Check sheet for the modelled part. Datum: model origin and axes. Units: mm. Face numbers are marked on the shaded views. A direction names the side the tool comes from. Round coordinates to 2 decimals unless told otherwise and drop trailing zeros. Order: outer loops, then holes, each group sorted by start corner. A loop starts at its lowest first (then second) coordinate and runs counter-clockwise, first axis right, second up.
(1) Sectioned sample at B-B, the plane x = 0. Enter the section's corners in (y, z).
(2) Tool access check on the marked faces 1, 2, 3, 4 and 5. Record the directions out of +Z, -Z, +X, -X, +Y, -Y that give a thin tool (end or side, any length) a straight path to the whole face; none if there is none.
(3) Depth check by flat-ended pin: pin 1 (2 mm diameter, centred on x = -1, z = -1.5, fed in from -Y); pin 2 (0.6 mm diameter, centred on x = -0.5, y = 1, fed in from +Z). Enter the tip coordinate at first touch or a pass-through.
(4) Thickness scan on probe 1 along Z at (x, y) = (0.7, -1); probe 2 along Z at (x, y) = (-2.4, -3); probe 3 along Y at (x, z) = (2.1, 4). Record the ranges inside material, lowest first.
(5) Sectioned sample at C-C, the plane y = 1.75. Enter the section's corners in (x, z), and give its area (3 significant figures).
(6) Sectioned sample at A-A, the plane z = 0. Enter the section's corners in (x, y).
(7) Sectioned sample at D-D, the plane z = 2. Enter the section's corners in (x, y), and give its area (3 significant figures).
```python
from build123d import *

# Parameters (mm, degrees)
SKETCH1_W           = 6
SKETCH1_H           = 6.95
BOSS_EXTRUDE1_DEPTH = 1.95
SKETCH2_R           = 2.5
BOSS_EXTRUDE2_DEPTH = 1.7
SKETCH3_W           = 6
SKETCH3_H           = 0.5
BOSS_EXTRUDE3_DEPTH = 1
SKETCH4_W           = 6
SKETCH4_H           = 0.5
BOSS_EXTRUDE4_DEPTH = 6


with BuildPart() as part:
    # Sketch1 → Boss-Extrude1 (new, symmetric)
    with BuildSketch(Plane(origin=(0, 0, 0), x_dir=(1, 0, 0), z_dir=(0, 1, 0))):
        with Locations((0, -0.825)):
            Rectangle(SKETCH1_W, SKETCH1_H)
    extrude(amount=BOSS_EXTRUDE1_DEPTH, both=True)

    # Sketch2 → Boss-Extrude2 (add)
    with BuildSketch(Plane(origin=(0, 1.95, 0), x_dir=(1, 0, 0), z_dir=(0, 1, 0))):
        with Locations(Location((0, 0, 0), (0, 0, 270))):
            Circle(SKETCH2_R)
    extrude(amount=BOSS_EXTRUDE2_DEPTH)

    # Sketch3 → Boss-Extrude3 (add)
    with BuildSketch(Plane.XY.offset(4.3)):
        with Locations((0, -0.25)):
            Rectangle(SKETCH3_W, SKETCH3_H)
    extrude(amount=BOSS_EXTRUDE3_DEPTH)

    # Sketch4 → Boss-Extrude4 (add)
    with BuildSketch(Plane.XZ.offset(0.5)):
        with Locations((0, 5.05)):
            Rectangle(SKETCH4_W, SKETCH4_H)
    extrude(amount=BOSS_EXTRUDE4_DEPTH)


solid = part.part
```
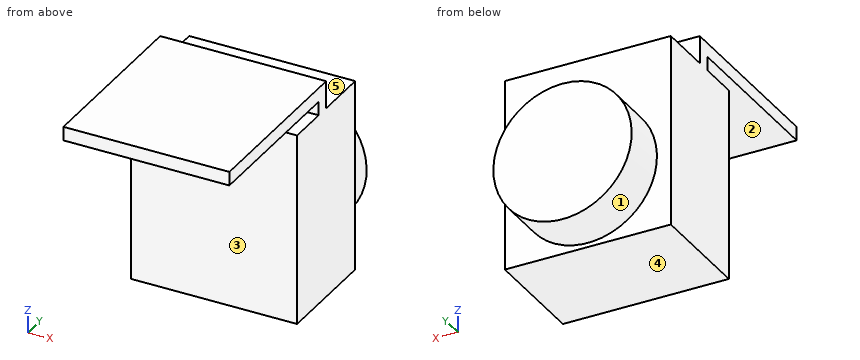
Derived:
1. outline: (-6.5, 4.8) - (-0.5, 4.8) - (-0.5, 4.3) - (-1.95, 4.3) - (-1.95, -2.65) - (1.95, -2.65) - (1.95, -2.5) - (3.65, -2.5) - (3.65, 2.5) - (1.95, 2.5) - (1.95, 4.3) - (0, 4.3) - (0, 5.3) - (-6.5, 5.3) - close
2. face 1: +Y
2. face 2: +X, -X, -Y
2. face 3: -Z, +X, -X, -Y
2. face 4: -Z, +X, -X, +Y, -Y
2. face 5: +Z, +X, -X, +Y
3. pin 1: stops at y = -1.95
3. pin 2: stops at z = 4.3
4. probe 1: z = -2.65 to 4.3, 4.8 to 5.3
4. probe 2: z = 4.8 to 5.3
4. probe 3: y = -1.95 to 1.95
5. outline: (-3, -2.65) - (3, -2.65) - (3, 4.3) - (-3, 4.3) - close
5. area: 41.7 mm2
6. outline: (-3, -1.95) - (3, -1.95) - (3, 1.95) - (2.5, 1.95) - (2.5, 3.65) - (-2.5, 3.65) - (-2.5, 1.95) - (-3, 1.95) - close
7. outline: (-3, -1.95) - (3, -1.95) - (3, 1.95) - (1.5, 1.95) - (1.5, 3.65) - (-1.5, 3.65) - (-1.5, 1.95) - (-3, 1.95) - close
7. area: 28.5 mm2
